For this review, use the dimensioned drawing (mm, ordinates from the lowest corner) and the shaded views. A direction names the side the tool comes from. Round coordinates to 2 decimals unless told otherwise and drop trailing zeros. Order: outer loops, then holes, each group sorted by start corner. A loop starts at its lowest first (then second) coordinate and runs counter-clockwise, first axis right, second up. Notation, with made-up numbers: (-19.5, 24) - (6.5, 24) arc R12 ccw to (6.5, 38) - close; hole circle Ø11 at (-0.75, -29.75). An arc over 180 degrees is marked (long way). Write item = value, one per line.
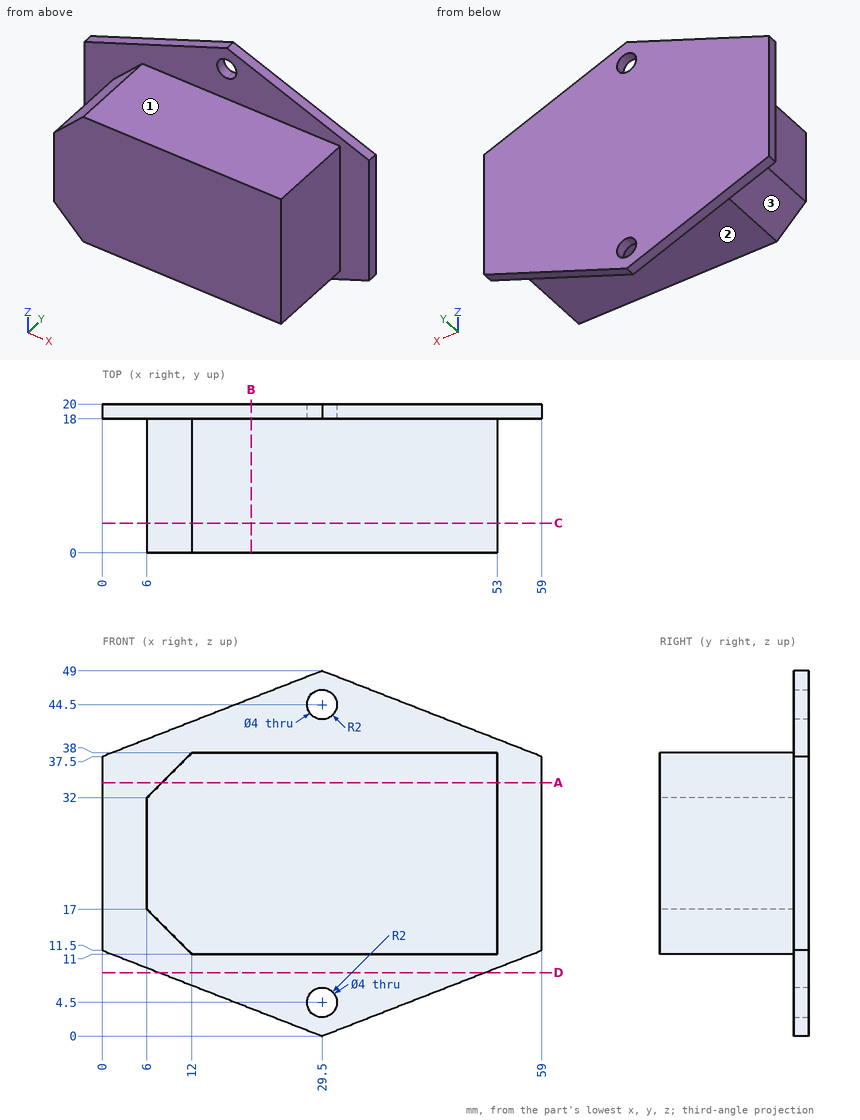
1) We need section B-B on x = 20. Write out the cut boundary in (y, z).
Findings:
outline = (0, 11) - (18, 11) - (18, 3.7) - (20, 3.7) - (20, 45.3) - (18, 45.3) - (18, 38) - (0, 38) - close
2) We need section A-A on z = 34. Write out the cut boundary in (x, y).
Findings:
outline = (0, 18) - (8, 18) - (8, 0) - (53, 0) - (53, 18) - (59, 18) - (59, 20) - (0, 20) - close
3) We need section D-D on z = 8.5. Write out the cut boundary in (x, y), and give its area (3 significant figures).
Findings:
outline = (7.7, 18) - (51.3, 18) - (51.3, 20) - (7.7, 20) - close
area = 87.2 mm^2
4) We need section C-C on y = 4. Write out the cut boundary in (x, z).
Findings:
outline = (6, 17) - (12, 11) - (53, 11) - (53, 38) - (12, 38) - (6, 32) - close
5) To check wall thickness, follow L1, parallel to Z at x = 29.5, y = 18.45; L2, parallel to X at y = 15.5, z = 17.5; L3, parallel to Z at x = 25.5, y = 13.5. State the ranges of each line that lie inside material, in increasing order. Write a range as from..to.
Findings:
L1 = 0..2.5, 6.5..42.5, 46.5..49
L2 = 6..53
L3 = 11..38
6) For the marked faces 1, 2 and 3, list the 3-axis set-ups (+Z, -Z, +X, -X, +Y, -Y) from which the entire face can be reached by the end or side of a thin tool; tool diameter is ignored.
Findings:
face_1 = +Z, +X, -X, -Y
face_2 = -Z, +X, -X, -Y
face_3 = -Z, -X, -Y
7) Clearance check with flat-ended pins moving along their axes: pin 1 Ø3.5 at (x, z) = (29.5, 44.5) entering from -Y; pin 2 Ø6 at (y, z) = (14, 35.5) entering from -X; pin 3 Ø6 at (x, y) = (35.5, 8.5) entering from +Z; pin 4 Ø12 at (y, z) = (7, 27.5) entering from -X. State where each tip first meets the part, or that it passes through.
Findings:
pin_1 = through
pin_2 = 6.5
pin_3 = 38
pin_4 = 6
